Geometry check sheet. Reference: the model listing, model coordinates, mm. Face numbers are marked on the shaded views. A direction names the side the tool comes from. Give positions to 0.01 mm unless a question says otherwise; leave off trailing zeros. Order: outer loops, then holes, each group sorted by start corner. A loop starts at its lowest first (then second) coordinate and runs counter-clockwise, first axis right, second up. Notation, with made-up numbers: M 82.5,76 L 134.5,76 A24 ccw 134.5,112 Z; hole C 64,28.5 d5. An arc over 180 degrees is marked long. Answer as CSV lines item,"result".
from build123d import *

# Parameters (mm, degrees)
F0_R     = 6.35
F1_DEPTH = 12.7
F2_R     = 25.4
F2_R_2   = 19.05
F3_DEPTH = 76.2
F4_SIZE  = 5.08


with BuildPart() as f1:
    # F0 (on Top) → F1 (new body)
    with BuildSketch(Plane.XY):
        with BuildLine():
            ThreePointArc((-66.04, -25.4), (-42.772685, -29.877305), (-21.514457, -40.341623))
            ThreePointArc((-21.514457, -40.341623), (0.226525, -45.719439), (21.913151, -40.126453))
            ThreePointArc((21.913151, -40.126453), (42.996249, -29.825744), (66.04, -25.4))
            ThreePointArc((66.04, -25.4), (91.44, 0), (66.04, 25.4))
            ThreePointArc((66.04, 25.4), (42.996249, 29.825744), (21.913151, 40.126453))
            ThreePointArc((21.913151, 40.126453), (0.226525, 45.719439), (-21.514457, 40.341623))
            ThreePointArc((-21.514457, 40.341623), (-42.772685, 29.877305), (-66.04, 25.4))
            ThreePointArc((-66.04, 25.4), (-91.44, 0), (-66.04, -25.4))
        make_face()
        with Locations((-66.04, 0)):
            Circle(F0_R, mode=Mode.SUBTRACT)
        with Locations((66.04, 0)):
            Circle(F0_R, mode=Mode.SUBTRACT)
    extrude(amount=F1_DEPTH)

    # F2 (on Top) → F3 (join)
    with BuildSketch(Plane.XY):
        Circle(F2_R)
        Circle(F2_R_2, mode=Mode.SUBTRACT)
    extrude(amount=F3_DEPTH)

    # F4
    f4_edges = [f1.edges().sort_by_distance(p)[0] for p in [
        (-19.05, 0, 76.2),
    ]]
    chamfer(f4_edges, length=F4_SIZE)


solid = f1.part
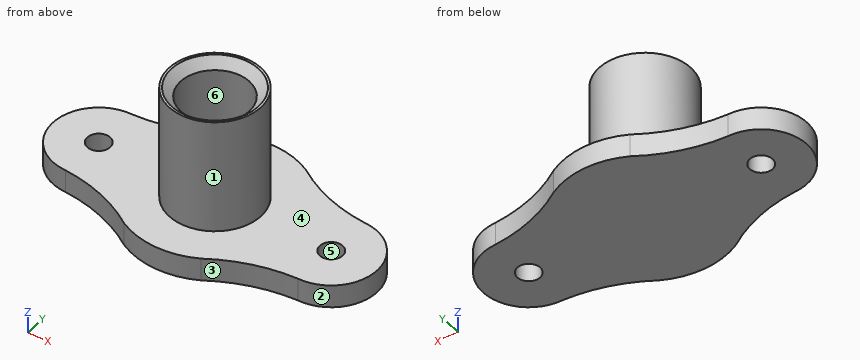
(1) Gauge pin test, flat ends, axial feed: P1, Ø3, axis at x = -50, y = 18.5, coming from the +Z side; P2, Ø12, axis at x = -36.5, z = 8, coming from the -Y side; P3, Ø20.5, axis at x = 66.04, y = 0, coming from the -Z side; P4, Ø6, axis at y = 18.5, z = 36.5, coming from the +X side. Record the tip position at first contact, or that the pin passes through.
The answers:
P1,"stops at z = 12.7"
P2,"stops at y = -35.05"
P3,"stops at z = 0"
P4,"stops at x = 20.12"
(2) Section check D-D on y = 28. Enter the section's corners in (x, z).
The answers:
outline,"M -49.15,0 L 49.21,0 L 49.21,12.7 L -49.15,12.7 Z"
(3) Tool access check on the marked faces 1 and 2. Record the directions out of +Z, -Z, +X, -X, +Y, -Y that give a thin tool (end or side, any length) a straight path to the whole face; none if there is none.
The answers:
face 1,"+Z"
face 2,"+Z, -Z, +X"
(4) Section check A-A on y = 0. Enter the section's corners in (x, z), then the cut area to 3 significant figures.
The answers:
outline,"M -91.44,0 L -72.39,0 L -72.39,12.7 L -91.44,12.7 Z; M -59.69,0 L 59.69,0 L 59.69,12.7 L 25.4,12.7 L 25.4,76.2 L 24.13,76.2 L 19.05,71.12 L 19.05,12.7 L -19.05,12.7 L -19.05,71.12 L -24.13,76.2 L -25.4,76.2 L -25.4,12.7 L -59.69,12.7 Z; M 72.39,0 L 91.44,0 L 91.44,12.7 L 72.39,12.7 Z"
area,"2,780 mm2"
(5) Section check C-C on z = 28.5. Enter the section's corners in (x, y).
The answers:
outline,"C 0,0 d50.8; hole C 0,0 d38.1"
(6) Section check B-B on x = 0. Enter the section's corners in (y, z), then the cut area to 3 significant figures.
The answers:
outline,"M -45.72,0 L 45.72,0 L 45.72,12.7 L 25.4,12.7 L 25.4,76.2 L 24.13,76.2 L 19.05,71.12 L 19.05,12.7 L -19.05,12.7 L -19.05,71.12 L -24.13,76.2 L -25.4,76.2 L -25.4,12.7 L -45.72,12.7 Z"
area,"1,940 mm2"
(7) Draft check along X on the marked faces 3, 4, 5 and 6. Enter one of: +X half, -X half, draft (parallel to the pull), parting line (faces both ways), or undercut.
The answers:
face 3,"+X half"
face 4,"draft"
face 5,"undercut"
face 6,"undercut"
(8) Material ranges on line 1 (X direction, y = 0, z = 34); line 2 (Z direction, x = 43, y = 7.5); line 3 (Y direction, x = 66, z = 4), recorded low to high.
The answers:
line 1,"x = -25.4 to -19.05, 19.05 to 25.4"
line 2,"z = 0 to 12.7"
line 3,"y = -25.4 to -6.35, 6.35 to 25.4"
